from build123d import *

# Parameters (mm, degrees)
F0_W     = 292.1
F0_H     = 539.75
F1_DEPTH = 19.05
F3_DEPTH = 19.05


with BuildPart() as f1:
    # F0 (on Right) → F1 (new body)
    with BuildSketch(Plane.YZ):
        with Locations((146.05, 269.875)):
            Rectangle(F0_W, F0_H)
    extrude(amount=F1_DEPTH)

    # F2 (on face) → F3 (cut)
    with BuildSketch(Plane.YZ.offset(19.05)):
        with BuildLine():
            Line((146.05, 25.4), (88.9, 25.4))
            ThreePointArc((88.9, 25.4), (70.939488, 17.960512), (63.5, 0))
            Line((63.5, 0), (228.6, 0))
            ThreePointArc((228.6, 0), (221.160512, 17.960512), (203.2, 25.4))
            Line((203.2, 25.4), (146.05, 25.4))
        make_face()
    extrude(amount=-F3_DEPTH, mode=Mode.SUBTRACT)


solid = f1.part
Verification items for the finished model (mm, model axes). A direction names the side the tool comes from. Coordinates: 2 decimals unless noted, no trailing zeros. Loops run counter-clockwise (first coordinate to the right, second up) from the corner with the lowest first, then second, coordinate; pieces in that order, holes last. Notation, with made-up numbers: M -10,29 L 36,29 A31 cw 36,59 Z; hole C 2,75.5 d10. An arc over 180 degrees is marked long. One line per item, written item: value.
1. Gauge pin test, flat ends, axial feed: P1, Ø9.5, axis at x = 6, y = 124, coming from the -Z side; P2, Ø1, axis at x = 10, y = 219.5, coming from the -Z side. Record the tip position at first contact, or that the pin passes through.
Answers follow:
P1: z = 25.4
P2: z = 19.05
2. Section check C-C on y = 72. Record the cut outline in (x, z), plus the area to 3 significant figures.
Answers follow:
outline: M 0,18.96 L 19.05,18.96 L 19.05,539.75 L 0,539.75 Z
area: 9,920 mm^2
3. Section check A-A on x = 14.75. Record the cut outline in (y, z), plus the area to 3 significant figures.
Answers follow:
outline: M 0,0 L 63.5,0 A25.4 cw 88.9,25.4 L 203.2,25.4 A25.4 cw 228.6,0 L 292.1,0 L 292.1,539.75 L 0,539.75 Z
area: 154,000 mm^2
4. Set-up check for faces 1 (the flat face through (0, 144, 274)), 2 (the cylindrical face through (9.66, 221.36, 17.76)): record each of +Z, -Z, +X, -X, +Y, -Y from which the full face is reachable in a straight line by a thin tool's end or side.
Answers follow:
face 1: +Z, -Z, -X, +Y, -Y
face 2: -Z, +X, -X
5. Material ranges on line 1 along Z through (x, y) = (16.25, 150); line 2 along Z through (x, y) = (16.25, 206.5), recorded low to high. Write a range as from..to.
Answers follow:
line 1: 25.4..539.75
line 2: 25.18..539.75
6. Mould release check, pull along Y, two halves, no side actions. Record for faces 3 (the flat face through (9, 292.1, 266)), 4 (the flat face through (10, 147, 25.4)), 5 (the flat face through (9, 0, 266)), 6 (the flat face through (9, 260, 0)): pulls with the +Y half, pulls with the -Y half, needs draft (parallel to the pull), parting line crosses it, or undercut.
Answers follow:
face 3: pulls with the +Y half
face 4: undercut
face 5: pulls with the -Y half
face 6: needs draft
7. Section check B-B on y = 120.5. Record the cut outline in (x, z).
Answers follow:
outline: M 0,25.4 L 19.05,25.4 L 19.05,539.75 L 0,539.75 Z
